```python
from build123d import *

# Parameters (mm, degrees)
CUT_EXTRUDE_1_DEPTH = 3
FILLET_1_R          = 0.3
CHAMFER_1_SIZE      = 1


with BuildPart() as part:
    # Эскиз1 → Повернуть1 (revolve)
    with BuildSketch(Plane.XY, mode=Mode.PRIVATE) as revolve_1_sk:
        Polygon((0, 0), (0, 5.9), (0.5, 5.9), (4, 3), (12, 3), (12, 0), align=None)
    revolve(revolve_1_sk.sketch.rotate(Axis((0, 0, 0), (1, 0, 0)), 90), axis=Axis((0, 0, 0), (1, 0, 0)))  # turned: the seam where the file's is

    # Эскиз2 → Вырез-Вытянуть1 (cut)
    with BuildSketch(Plane.ZY):
        Polygon((1.154700538, 2), (-1.154700538, 2), (-2.309401077, 0), (-1.154700538, -2), (1.154700538, -2), (2.309401077, 0), align=None)
    extrude(amount=-CUT_EXTRUDE_1_DEPTH, mode=Mode.SUBTRACT)

    # Скругление1
    fillet_1_edges = [part.edges().sort_by_distance(p)[0] for p in [
        (0, 0, -5.9),
    ]]
    fillet(fillet_1_edges, radius=FILLET_1_R)

    # Фаска1
    chamfer_1_edges = [part.edges().sort_by_distance(p)[0] for p in [
        (12, 0, -3),
    ]]
    chamfer(chamfer_1_edges, length=CHAMFER_1_SIZE)


solid = part.part
```
Here's how the part is built. I have some questions about the finished solid (model axes, mm). A direction names the side the tool comes from. Round coordinates to 2 decimals unless told otherwise and drop trailing zeros. Order: outer loops, then holes, each group sorted by start corner. A loop starts at its lowest first (then second) coordinate and runs counter-clockwise, first axis right, second up. Notation, with made-up numbers: M 87,1.25 L 115,1.25 A5 ccw 115,9.25 Z; hole C 46.25,-10.75 d9. An arc over 180 degrees is marked long. One line per question, with ' | ' between items.
1) I want a section at A-A, the plane x = 2. Write out the boundary of the cut face in (y, z), then the cut area to 3 significant figures.
Working result:
outline: C 0,0 d9.31; hole M -2,-1.15 L 0,-2.31 L 2,-1.15 L 2,1.15 L 0,2.31 L -2,1.15 Z | area: 54.3 mm²
2) I want a section at B-B, the plane z = 0. Write out the boundary of the cut face in (x, y), then the cut area to 3 significant figures.
Working result:
outline: M 0,-5.6 A0.3 ccw 0.3,-5.9 L 0.5,-5.9 L 4,-3 L 11,-3 L 12,-2 L 12,2 L 11,3 L 4,3 L 0.5,5.9 L 0.3,5.9 A0.3 ccw 0,5.6 L 0,2 L 3,2 L 3,-2 L 0,-2 Z | area: 72.0 mm²
3) For pin 1 Ø4 at (x, y) = (10, -1.5) entering from +Z; pin 2 Ø0.7 at (x, z) = (1, 0) entering from -Y; pin 3 Ø4 at (y, z) = (4, 2.5) entering from +X, each with a flat end and sliding along its axis, tell me the tip position at first contact or that it passes through.
Working result:
pin 1: z = 3 | pin 2: y = -5.78 | pin 3: x = 11.28
4) For faces 4 (the face through (1.48, 0.99, 1.74)), 5 (the face through (3.83, -0.943, 2.996)), which set-ups out of +Z, -Z, +X, -X, +Y, -Y let a thin tool reach every point of the face, with its end or its side?
Working result:
face 4: -X | face 5: +X
5) If we mould it in two halves opening along Z, with no side actions, what happens to faces 1 (the face through (7.55, -0.9, 2.86)), 2 (the face through (12, 0, 0)), 3 (the face through (1.48, -0.99, -1.74))? For each: +Z half, -Z half, draft (parallel to the pull), parting line (faces both ways), or undercut.
Working result:
face 1: parting line | face 2: draft | face 3: undercut
6) I want a section at C-C, the plane x = 10.25. Write out the boundary of the cut face in (y, z).
Working result:
outline: C 0,0 d6
7) I need wall thicknesses on line 1 along X through (y, z) = (-1.5, -1.25); line 2 along Y through (x, z) = (1.5, -0.75); line 3 along Y through (x, z) = (6.5, 1.75). Which ranges of each line are inside material? Lowest first, please.
Working result:
line 1: 3 to 12 | line 2: -5.02 to -2, 2 to 5.02 | line 3: -2.44 to 2.44
